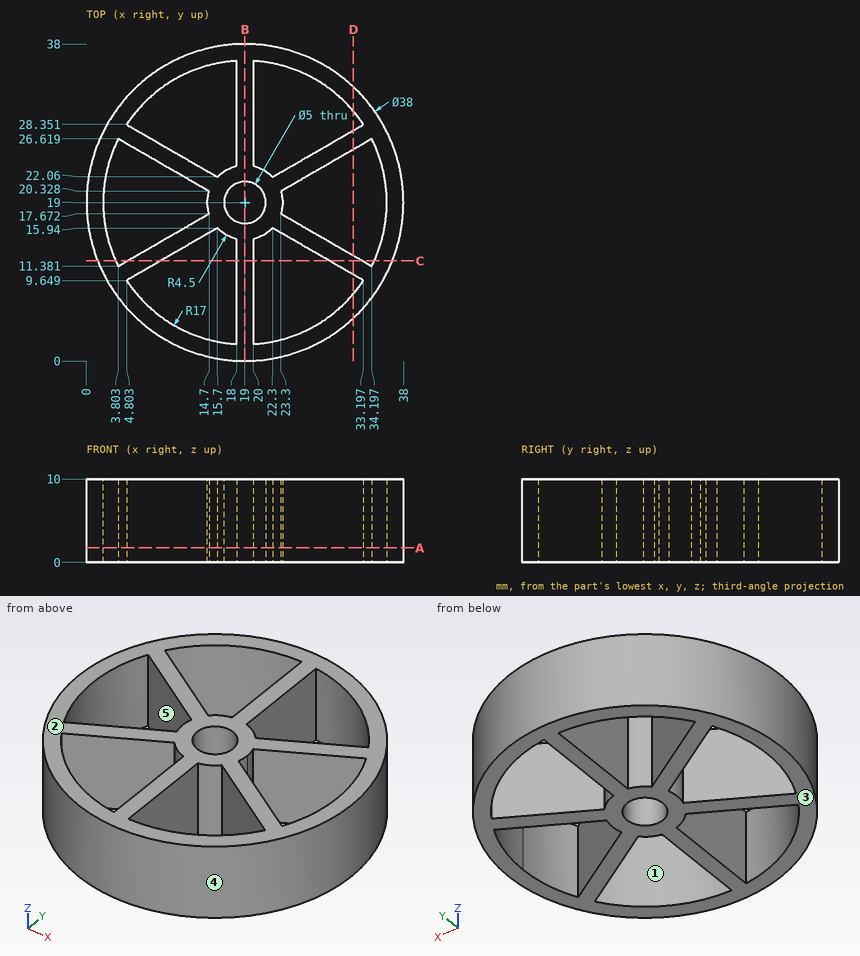
Input: dimensioned drawing with shaded views. Units: mm. Origin: part minimum x, y, z. A direction names the side the tool comes from. Coordinates: 2 decimals unless noted, no trailing zeros. Loops run counter-clockwise (first coordinate to the right, second up) from the corner with the lowest first, then second, coordinate; pieces in that order, holes last. Notation, with made-up numbers: M -6,2 L 44,2 A32 ccw 44,40 Z; hole C 14,22.5 d1. An arc over 180 degrees is marked long. Use a Markdown table: item, result. Add a question column.
1) Line query: L1, parallel to X at y = 13.5, z = 3.25 (1 decimal); L2, parallel to X at y = 15, z = 4.25 (1 decimal); L3, parallel to Y at x = 19, z = 3.75. Output: solid intervals per line, ascending. Write a range as from..to.
2) Set-up query: the marked faces 1 and 2. Return all of +Z, -Z, +X, -X, +Y, -Y with unobstructed straight access to the full face (end or side cutting, diameter ignored); none if empty.
3) Section B-B, the plane x = 19. Return the cut outline in (y, z).
4) Section D-D, the plane x = 32. Return the cut outline in (y, z) (1 decimal).
5) Section A-A, the plane z = 1.75. Return the cut outline in (x, y).
6) Draft query along Y for the marked faces 3, 4 and 5. Return one class per face: +Y half, -Y half, draft (parallel to the pull), parting line (faces both ways), or undercut.
7) Pin query (flat end, axial travel): P1, Ø8, axis at x = 23.5, y = 24, coming from the +Z side; P2, Ø1, axis at x = 15.5, z = 5, coming from the +Y side; P3, Ø1, axis at y = 20, z = 7.5, coming from the -X side; P4, Ø3, axis at y = 30.5, z = 6, coming from the +X side (1 decimal). Return the tip coordinate at first contact, or that it passes through.
8) Section C-C, the plane y = 12. Return the cut outline in (x, z) (1 decimal).
Answer below:
| question | item | result |
|---|---|---|
| 1 | L1 | 0.8..2.9, 7.5..11.5, 18..20, 26.5..30.5, 35.1..37.2 |
| 1 | L2 | 0.4..2.5, 10.1..14.1, 16.9..21.1, 23.9..27.9, 35.5..37.6 |
| 1 | L3 | 0..16.5, 21.5..38 |
| 2 | face 1 | +Z, -Z |
| 2 | face 2 | +Z, +X, -X, +Y, -Y |
| 3 | outline | M 0,0 L 16.5,0 L 16.5,10 L 0,10 Z; M 21.5,0 L 38,0 L 38,10 L 21.5,10 Z |
| 4 | outline | M 5.1,0 L 8,0 L 8,10 L 5.1,10 Z; M 10.3,0 L 12.6,0 L 12.6,10 L 10.3,10 Z; M 25.4,0 L 27.7,0 L 27.7,10 L 25.4,10 Z; M 30,0 L 32.9,0 L 32.9,10 L 30,10 Z |
| 5 | outline | C 19,19 d38; hole M 3.8,11.38 L 14.7,17.67 A4.5 cw 14.7,20.33 L 3.8,26.62 A17 ccw Z; hole M 4.8,9.65 A17 ccw 18,2.03 L 18,14.61 A4.5 cw 15.7,15.94 Z; hole M 4.8,28.35 L 15.7,22.06 A4.5 cw 18,23.39 L 18,35.97 A17 ccw Z; hole C 19,19 d5; hole M 20,2.03 A17 ccw 33.2,9.65 L 22.3,15.94 A4.5 cw 20,14.61 Z; hole M 20,23.39 A4.5 cw 22.3,22.06 L 33.2,28.35 A17 ccw 20,35.97 Z; hole M 23.3,17.67 L 34.2,11.38 A17 ccw 34.2,26.62 L 23.3,20.33 A4.5 cw Z |
| 6 | face 3 | draft |
| 6 | face 4 | parting line |
| 6 | face 5 | undercut |
| 7 | P1 | z = 10 |
| 7 | P2 | y = 37.76 |
| 7 | P3 | x = 0.01 |
| 7 | P4 | x = 35.2 |
| 8 | outline | M 1.3,0 L 3.5,0 L 3.5,10 L 1.3,10 Z; M 4.9,0 L 8.9,0 L 8.9,10 L 4.9,10 Z; M 18,0 L 20,0 L 20,10 L 18,10 Z; M 29.1,0 L 33.1,0 L 33.1,10 L 29.1,10 Z; M 34.5,0 L 36.7,0 L 36.7,10 L 34.5,10 Z |
